from build123d import *

# Parameters (mm, degrees)
F0_R           = 4
F1_DEPTH       = 80
F4_D           = 2.4
F4_DEPTH       = 50
F4_CSINK_D     = 6.72
F4_CSINK_ANGLE = 90
F4_TIP         = 0.7210327428
F5_ANGLE       = 180


with BuildPart() as f1:
    # F0 (on Top) → F1 (new body)
    with BuildSketch(Plane.XY):
        Circle(F0_R)
    extrude(amount=F1_DEPTH)

    # F4
    with Locations(Plane(origin=(0, 4, 0), x_dir=(1, 0, 0), z_dir=(0, 1, 0))):
        with Locations((0, -55), (0, -25)):
            CounterSinkHole(F4_D / 2, F4_CSINK_D / 2, depth=F4_DEPTH, counter_sink_angle=F4_CSINK_ANGLE)
            with Locations((0, 0, -(F4_DEPTH + F4_TIP / 2))):  # 118° drill point
                Cone(0, F4_D / 2, F4_TIP, mode=Mode.SUBTRACT)


with BuildPart() as f1_1:
    # F5: moved
    add(f1.part.rotate(Axis((0, 0, 80), (0, 0, 1)), F5_ANGLE))


solid = f1_1.part
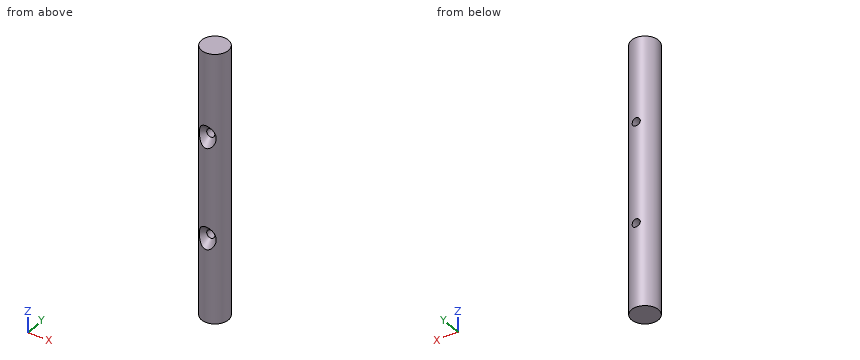
Here's how the part is built. I have some questions about the finished solid (model axes, mm). Give positions to 0.01 mm unless a question says otherwise; leave off trailing zeros. Loops run counter-clockwise (first coordinate to the right, second up) from the corner with the lowest first, then second, coordinate; pieces in that order, holes last. Notation, with made-up numbers: (-14, -7.5) -> (19, -7.5) arc R25 cw to (19, 15.5) -> close; hole circle Ø3 at (58, 30). An arc over 180 degrees is marked (long way). One line per item, written item: value.
Q1. Suppose I cut it at B-B on z = 25. Please give me the cut outline in (x, y).
Answers follow:
outline: (-2.49, -3.13) -> (-1.2, -1.84) -> (-1.2, 3.82) arc R4 ccw to start; (1.2, -1.84) -> (2.49, -3.13) arc R4 ccw to (1.2, 3.82) -> close
Q2. Suppose I cut it at A-A on x = 0. Please give me the cut outline in (y, z).
Answers follow:
outline: (-4, 0) -> (4, 0) -> (4, 23.8) -> (-1.84, 23.8) -> (-4, 21.64) -> close; (-4, 28.36) -> (-1.84, 26.2) -> (4, 26.2) -> (4, 53.8) -> (-1.84, 53.8) -> (-4, 51.64) -> close; (-4, 58.36) -> (-1.84, 56.2) -> (4, 56.2) -> (4, 80) -> (-4, 80) -> close
Q3. I'm going to push flat-ended pins straight in: pin 1 Ø2 at (y, z) = (-3, 13) entering from -X; pin 2 Ø3 at (x, z) = (-2.5, 54) entering from +Y. Where does each tip first touch, or does it pass through?
Answers follow:
pin 1: x = -3.46
pin 2: y = 3.87
Q4. If I drill on line 1 along Z through (x, y) = (0, 0.8); line 2 along X through (y, z) = (0.1, 55); line 3 along Z through (x, y) = (0.5, 1.25), over which ranges is the centre line in solid material (lowest first)?
Answers follow:
line 1: 0 to 23.8, 26.2 to 53.8, 56.2 to 80
line 2: -4 to -1.2, 1.2 to 4
line 3: 0 to 23.91, 26.09 to 53.91, 56.09 to 80
Q5. Suppose I cut it at D-D on z = 50. Please give me the cut outline in (x, y).
Answers follow:
outline: circle Ø8 at (0, 0)
Q6. Suppose I cut it at C-C on y = 1.5. Please give me the cut outline in (x, z), then the cut area to 3 significant figures.
Answers follow:
outline: (-3.71, 0) -> (3.71, 0) -> (3.71, 80) -> (-3.71, 80) -> close; hole circle Ø2.4 at (0, 25); hole circle Ø2.4 at (0, 55)
area: 584 mm^2
